Could you check a few things on this model? Use its own coordinates, in mm. A direction names the side the tool comes from. Give positions to 0.01 mm unless a question says otherwise; leave off trailing zeros. Order: outer loops, then holes, each group sorted by start corner. A loop starts at its lowest first (then second) coordinate and runs counter-clockwise, first axis right, second up. Notation, with made-up numbers: (60.25, 78.25) - (66.25, 78.25) arc R21 ccw to (66.25, 106.25) - close; hole circle Ø4 at (-31, 48.25). An arc over 180 degrees is marked (long way). One line per question, with ' | ' between items. Start each with the question number.
1. Imagine slicing it at A-A (y = 68). Please give me the cut outline in (x, z), and give its area (3 significant figures).
2. I need wall thicknesses on probe 1 along Z at (x, y) = (18.55, 111.76); probe 2 along X at (y, z) = (13.5, -1.5); probe 3 along Y at (x, z) = (4, 6.5). Which ranges of each line are inside material? Lowest first, please. Write a range as from..to.
3. Imagine slicing it at D-D (x = -1). Please give me the cut outline in (y, z).
4. Imagine slicing it at C-C (z = 10.5). Please give me the cut outline in (x, y), and give its area (3 significant figures).
5. Imagine slicing it at B-B (z = 5). Please give me the cut outline in (x, y).
6. Which directions (+Z, -Z, +X, -X, +Y, -Y) give clear straight access to the entire face, cutting with the end or side of a thin tool? Please do faces 5 (the flat face through (16.51, 63, 0)), 6 (the cylindrical face through (-18.06, -1.61, -0.18)).
7. If we mould it in two halves opening along Z, with no side actions, what happens to faces 1 (the flat face through (17, 42, 12.7)), 2 (the flat face through (-16.51, 63, 0)), 3 (the flat face through (17, 42, -12.7)), 4 (the cylindrical face through (17.798, 115.174, 5.354))? For each: released by +Z, released by -Z, zero draft, split by the parting line, or undercut.
8. For P1, Ø7.5, axis at x = 7.5, z = -0.5, coming from the +Y side, with a flat end and sliding along its axis, tell me the tip position at first contact or that it passes through.
```python
from build123d import *

# Parameters (mm, degrees)
SKETCH2_W                      = 38.1
SKETCH2_H                      = 25.4
BASE_FLANGE1_DEPTH             = 2.54
EDGE_FLANGE1_STRIP_W           = 11.6332
EDGE_FLANGE1_STRIP_H           = 2.54
EDGE_FLANGE1_STRIP_CUT_DEPTH   = 25.4
EDGE_FLANGE1_STRIP_2_W         = 11.6332
EDGE_FLANGE1_STRIP_2_H         = 2.54
EDGE_FLANGE1_STRIP_CUT_2_DEPTH = 25.4
EDGE_FLANGE1_DEPTH             = 25.4
EDGE_FLANGE1_BEND_DEPTH        = 25.4
CUT_EXTRUDE1_DEPTH             = 131.779171124
SKETCH14_R                     = 6.35
CUT_EXTRUDE2_DEPTH             = 131.779171124


# Sheet-metal steps are written as plain solids
with BuildPart() as part:
    # Sketch2 → Base-Flange1 (new body)
    with BuildSketch(Plane(origin=(0, 0, 0), x_dir=(1, 0, 0), z_dir=(0, 1, 0))):
        Rectangle(SKETCH2_W, SKETCH2_H)
    extrude(amount=-BASE_FLANGE1_DEPTH)

    # Edge-Flange1 strip (across the edge) → Edge-Flange1 strip cut (cut)
    with BuildSketch(Plane(origin=(19.05, 0, 12.7), x_dir=(-1, 0, 0), z_dir=(0, 0, -1))):
        with Locations((-2.54, -1.27)):
            Rectangle(EDGE_FLANGE1_STRIP_W, EDGE_FLANGE1_STRIP_H)
    extrude(amount=EDGE_FLANGE1_STRIP_CUT_DEPTH, mode=Mode.SUBTRACT)

    # Edge-Flange1 strip 2 (across the edge) → Edge-Flange1 strip cut 2 (cut)
    with BuildSketch(Plane(origin=(-19.05, 0, -12.7), x_dir=(1, 0, 0), z_dir=(0, 0, 1))):
        with Locations((-2.54, -1.27)):
            Rectangle(EDGE_FLANGE1_STRIP_2_W, EDGE_FLANGE1_STRIP_2_H)
    extrude(amount=EDGE_FLANGE1_STRIP_CUT_2_DEPTH, mode=Mode.SUBTRACT)

    # Edge-Flange1 section (across the edge) → Edge-Flange1 (add)
    with BuildSketch(Plane(origin=(19.05, 0, 12.7), x_dir=(-1, 0, 0), z_dir=(0, 0, -1))):
        with BuildLine():
            Line((0, 0.7366), (0, 124.46))
            Line((0, 124.46), (2.54, 124.46))
            Line((2.54, 124.46), (2.54, 0.7366))
            ThreePointArc((2.54, 0.7366), (2.755745145, 0.215745145), (3.2766, 0))
            Line((3.2766, 0), (3.2766, -2.54))
            ThreePointArc((3.2766, -2.54), (0.959693921, -1.580306079), (0, 0.7366))
        make_face()
    extrude(amount=EDGE_FLANGE1_DEPTH)

    # Edge-Flange1 section 2 (across the edge) → Edge-Flange1 bend (add)
    with BuildSketch(Plane(origin=(-19.05, 0, -12.7), x_dir=(1, 0, 0), z_dir=(0, 0, 1))):
        with BuildLine():
            Line((0, 0.7366), (0, 124.46))
            Line((0, 124.46), (2.54, 124.46))
            Line((2.54, 124.46), (2.54, 0.7366))
            ThreePointArc((2.54, 0.7366), (2.755745145, 0.215745145), (3.2766, 0))
            Line((3.2766, 0), (3.2766, -2.54))
            ThreePointArc((3.2766, -2.54), (0.959693921, -1.580306079), (0, 0.7366))
        make_face()
    extrude(amount=EDGE_FLANGE1_BEND_DEPTH)

    # Sketch13 → Cut-Extrude1 (cut, through all)
    with BuildSketch(Plane(origin=(19.05, 0, 0), x_dir=(0, 0, -1), z_dir=(1, 0, 0))):
        with BuildLine():
            ThreePointArc((-2.4e-08, 124.46), (8.980256112, 120.74025613), (12.7, 111.76))
            Line((12.7, 111.76), (12.7, 124.46))
            Line((12.7, 124.46), (-2.4e-08, 124.46))
        make_face()
        with BuildLine():
            Line((-12.7, 124.46), (-12.7, 111.76))
            ThreePointArc((-12.7, 111.76), (-8.98025613, 120.740256112), (-2.4e-08, 124.46))
            Line((-2.4e-08, 124.46), (-12.7, 124.46))
        make_face()
    extrude(amount=-CUT_EXTRUDE1_DEPTH, mode=Mode.SUBTRACT)

    # Sketch14 → Cut-Extrude2 (cut, through all)
    with BuildSketch(Plane(origin=(19.05, 0, 0), x_dir=(0, 0, -1), z_dir=(1, 0, 0))):
        with Locations(Location((0, 111.76, 0), (0, 0, 90))):
            Circle(SKETCH14_R)
    extrude(amount=-CUT_EXTRUDE2_DEPTH, mode=Mode.SUBTRACT)


solid = part.part
```
Results found:
1) outline: (-19.05, -12.7) - (-16.51, -12.7) - (-16.51, 12.7) - (-19.05, 12.7) - close; (16.51, -12.7) - (19.05, -12.7) - (19.05, 12.7) - (16.51, 12.7) - close | area: 129 mm2
2) probe 1: z = -12.7..-6.35, 6.35..12.7 | probe 2: x = -19.05..-16.51, 16.51..19.05 | probe 3: y = -2.54..0
3) outline: (-2.54, -12.7) - (0, -12.7) - (0, 12.7) - (-2.54, 12.7) - close
4) outline: (-19.05, 0.74) arc R3.28 ccw to (-15.77, -2.54) - (15.77, -2.54) arc R3.28 ccw to (19.05, 0.74) - (19.05, 118.9) - (16.51, 118.9) - (16.51, 0.74) arc R0.74 cw to (15.77, 0) - (-15.77, 0) arc R0.74 cw to (-16.51, 0.74) - (-16.51, 118.9) - (-19.05, 118.9) - close | area: 696 mm2
5) outline: (-19.05, 0.74) arc R3.28 ccw to (-15.77, -2.54) - (15.77, -2.54) arc R3.28 ccw to (19.05, 0.74) - (19.05, 107.85) - (16.51, 107.85) - (16.51, 0.74) arc R0.74 cw to (15.77, 0) - (-15.77, 0) arc R0.74 cw to (-16.51, 0.74) - (-16.51, 107.85) - (-19.05, 107.85) - close; (-19.05, 115.67) - (-16.51, 115.67) - (-16.51, 123.43) - (-19.05, 123.43) - close; (16.51, 115.67) - (19.05, 115.67) - (19.05, 123.43) - (16.51, 123.43) - close
6) face 5: +Z, -Z, +Y | face 6: +Z, -Z, -X, -Y
7) face 1: released by +Z | face 2: zero draft | face 3: released by -Z | face 4: undercut
8) P1: stops at y = 0
